The figure shows three views and two pictorial views of one solid part (mm, origin at its lowest corner). Answer the questions. Round coordinates to 2 decimals unless told otherwise and drop trailing zeros. Order: outer loops, then holes, each group sorted by start corner. A loop starts at its lowest first (then second) coordinate and runs counter-clockwise, first axis right, second up. Notation, with made-up numbers: (17, 70) - (68, 70) arc R23 cw to (68, 85) - close; hole circle Ø1 at (5.25, 14.5). An arc over 180 degrees is marked (long way). Write item = value, one per line.
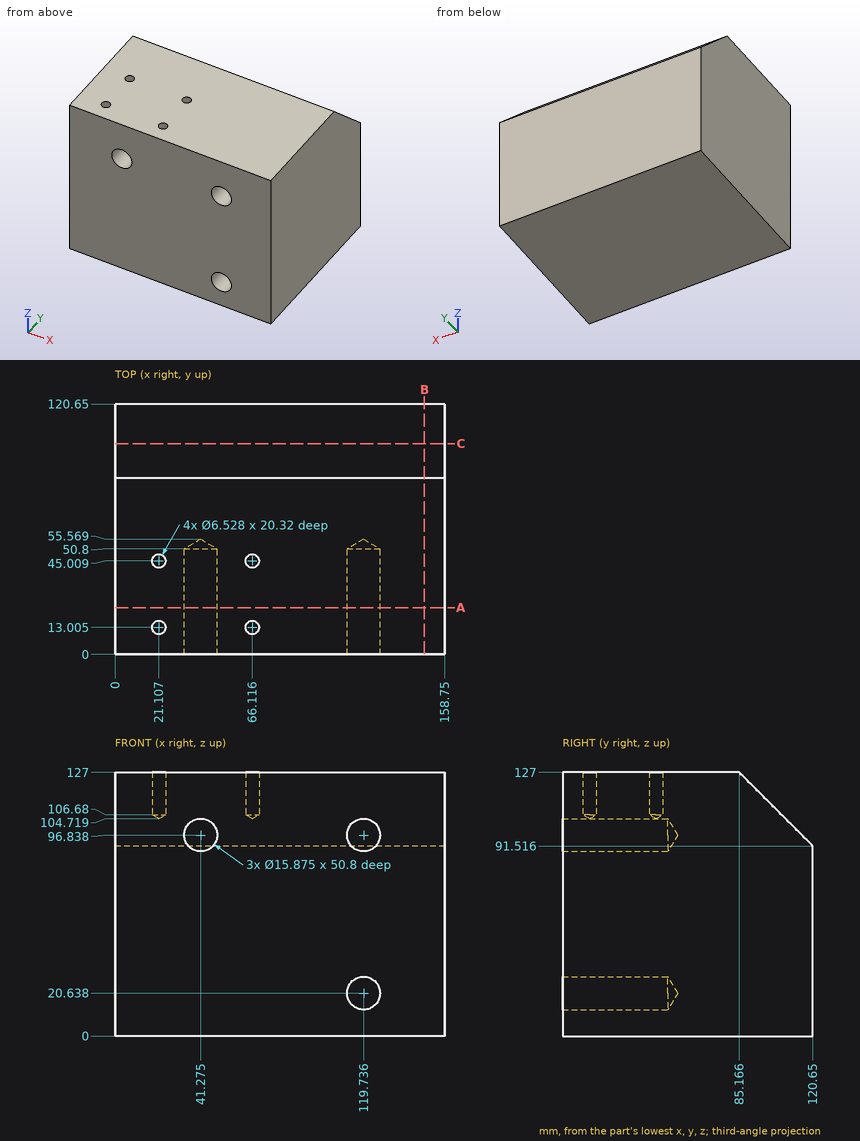
Q1. Section A-A on y = 22.5 is taken. Count the separate pieces of the cut face and the enclosed holes in it, then the cut area to 3 significant figures.
Model answer:
separate_pieces = 1
enclosed_holes = 3
area = 19,600 mm^2
Q2. Flat-ended cylindrical pins translate along their axes: P1, Ø5, axis at x = 66.12, y = 13, coming from the +Z side (1 decimal); P2, Ø9.5, axis at x = 41.28, z = 96.84, coming from the -Y side; P3, Ø8, axis at x = 23.5, y = 92, coming from the +Z side (1 decimal). Find the tip coordinate at first contact, or state that the pin passes through.
Model answer:
P1 = 106.2
P2 = 52.71
P3 = 124.2
Q3. Section B-B on x = 149 is taken. Determine the outline of the cut face in (y, z), then the cut area to 3 significant figures.
Model answer:
outline = (0, 0) - (120.65, 0) - (120.65, 91.52) - (85.17, 127) - (0, 127) - close
area = 14,700 mm^2
Q4. Section C-C on y = 101.5 is taken. Determine the outline of the cut face in (x, z).
Model answer:
outline = (0, 0) - (158.75, 0) - (158.75, 110.67) - (0, 110.67) - close
Q5. Find the intervals of material crossed by line 1 (X direction, y = 14, z = 20); line 2 (X direction, y = 7, z = 25.5); line 3 (Z direction, x = 151, y = 109.5) (1 decimal), in increasing order. Write a range as from..to.
Model answer:
line_1 = 0..111.82, 127.65..158.75
line_2 = 0..113.46, 126.01..158.75
line_3 = 0..102.7
